Read the model definition and answer for the solid it produces. Units are mm, in the model's axes. Face numbers are marked on the shaded views. A direction names the side the tool comes from. Give positions to 0.01 mm unless a question says otherwise; leave off trailing zeros. Order: outer loops, then holes, each group sorted by start corner. A loop starts at its lowest first (then second) coordinate and runs counter-clockwise, first axis right, second up.
Item 1: A cutting plane is placed at B-B (x = 4.5). Write down the section's boundary in (y, z) (3 decimals), plus the area to 3 significant figures.
Item 2: A cutting plane is placed at C-C (z = -6). Write down the section's boundary in (x, y) (3 decimals).
Item 3: The mould has two halves that part along Y. Classify the marked faces 1, 2 and 3: +Y half, -Y half, draft (parallel to the pull), parting line (faces both ways), or undercut.
Item 4: Which of the six approach directions +Z, -Z, +X, -X, +Y, -Y give full straight-line access (tool end or side, diameter ignored) to the marked faces 4 and 5?
Item 5: A cutting plane is placed at A-A (y = 9.5). Write down the section's boundary in (x, z) (3 decimals).
Item 6: Given pin 1 Ø4.5 at (x, y) = (-23.241, 23.241) entering from -Z (3 decimals); pin 2 Ø1.7 at (x, y) = (23, -18) entering from +Z; pin 3 Ø3.5 at (x, y) = (22.86, 17.78) entering from +Z; pin 4 Ø4.5 at (x, y) = (-23.241, -23.241) entering from +Z (3 decimals), each flat-ended and moving along its own axis, determine where each tip first touches the part or whether it passes through.
Item 7: Find the intervals of material crossed by line 1 along X through (y, z) = (27.5, 0) (3 decimals); line 2 along X through (y, z) = (7, -1) (3 decimals); line 3 along Y through (x, z) = (1.5, 6) (3 decimals), in increasing order.
Item 8: A cutting plane is placed at D-D (x = 12.7). State how many separate pieces and enclosed holes the cut face has, plus the area to 3 significant figures.
from build123d import *

# Parameters (mm, degrees)
SKETCH1_W_MOCK_PCB_W                      = 57.15
SKETCH1_W_MOCK_PCB_H                      = 57.15
BOSS_EXTRUDE1_DEPTH                       = 6.985
CUT_EXTRUDE1_DEPTH                        = 2.54
CUT_EXTRUDE3_DEPTH                        = 3.8608
F_4_40_TAPPED_HOLE1_AT_2_COUNT            = 2
F_4_40_TAPPED_HOLE1_AT_2_PITCH            = 45.72
F_4_40_TAPPED_HOLE1_AT_3_COUNT            = 2
F_4_40_TAPPED_HOLE1_AT_3_PITCH            = 35.56
F_4_40_TAPPED_HOLE1_AT_4_COUNT            = 2
F_4_40_TAPPED_HOLE1_AT_4_PITCH            = 57.920911595
F_4_40_TAPPED_HOLE2_AT_2_COUNT            = 2
F_4_40_TAPPED_HOLE2_AT_2_PITCH            = 46.482
F_4_40_TAPPED_HOLE2_AT_3_COUNT            = 2
F_4_40_TAPPED_HOLE2_AT_3_PITCH            = 65.735474806
F_4_40_TAPPED_HOLE2_AT_4_COUNT            = 2
F_4_40_TAPPED_HOLE2_AT_4_PITCH            = 46.482
F_8_32_TAPPED_HOLE1_D                     = 4.1656
F_8_32_TAPPED_HOLE1_DEPTH                 = 4.953
F_8_32_TAPPED_HOLE1_CSINK_D               = 4.191
F_8_32_TAPPED_HOLE1_CSINK_ANGLE           = 90
F_8_32_TAPPED_HOLE1_ON_FACE_2_D           = 4.1656
F_8_32_TAPPED_HOLE1_ON_FACE_2_DEPTH       = 4.953
F_8_32_TAPPED_HOLE1_ON_FACE_2_CSINK_D     = 4.191
F_8_32_TAPPED_HOLE1_ON_FACE_2_CSINK_ANGLE = 90


with BuildPart() as part:
    # Sketch1 w/mock PCB → Boss-Extrude1 (new body, symmetric)
    with BuildSketch(Plane.XY):
        Rectangle(SKETCH1_W_MOCK_PCB_W, SKETCH1_W_MOCK_PCB_H)
        with BuildLine():
            Line((20.32, 17.78), (20.32, 20.447))
            ThreePointArc((20.32, 20.447), (19.39006403, 22.69206403), (17.145, 23.622))
            Line((17.145, 23.622), (-17.145, 23.622))
            ThreePointArc((-17.145, 23.622), (-19.39006403, 22.69206403), (-20.32, 20.447))
            Line((-20.32, 20.447), (-20.32, 17.78))
            ThreePointArc((-20.32, 17.78), (-21.044102303, 16.004017017), (-22.803555556, 15.240627238))
            ThreePointArc((-22.803555556, 15.240627238), (-25.002872121, 14.286390014), (-25.908, 12.066411285))
            Line((-25.908, 12.066411285), (-25.908, -12.066411285))
            ThreePointArc((-25.908, -12.066411285), (-25.002872121, -14.286390014), (-22.803555556, -15.240627238))
            ThreePointArc((-22.803555556, -15.240627238), (-21.044102303, -16.004017017), (-20.32, -17.78))
            Line((-20.32, -17.78), (-20.32, -20.447))
            ThreePointArc((-20.32, -20.447), (-19.39006403, -22.69206403), (-17.145, -23.622))
            Line((-17.145, -23.622), (17.145, -23.622))
            ThreePointArc((17.145, -23.622), (19.39006403, -22.69206403), (20.32, -20.447))
            Line((20.32, -20.447), (20.32, -17.78))
            ThreePointArc((20.32, -17.78), (21.044102303, -16.004017017), (22.803555556, -15.240627238))
            ThreePointArc((22.803555556, -15.240627238), (25.002872121, -14.286390014), (25.908, -12.066411285))
            Line((25.908, -12.066411285), (25.908, 12.066411285))
            ThreePointArc((25.908, 12.066411285), (25.002872121, 14.286390014), (22.803555556, 15.240627238))
            ThreePointArc((22.803555556, 15.240627238), (21.044102303, 16.004017017), (20.32, 17.78))
        make_face(mode=Mode.SUBTRACT)
    extrude(amount=BOSS_EXTRUDE1_DEPTH, both=True)

    # Sketch2 → Cut-Extrude1 (cut)
    with BuildSketch(Plane.XY.offset(6.985)):
        with BuildLine():
            Line((-23.876, 27.051), (23.876, 27.051))
            ThreePointArc((23.876, 27.051), (26.12106403, 26.12106403), (27.051, 23.876))
            Line((27.051, 23.876), (27.051, -23.876))
            ThreePointArc((27.051, -23.876), (26.12106403, -26.12106403), (23.876, -27.051))
            Line((23.876, -27.051), (-23.876, -27.051))
            ThreePointArc((-23.876, -27.051), (-26.12106403, -26.12106403), (-27.051, -23.876))
            Line((-27.051, -23.876), (-27.051, 23.876))
            ThreePointArc((-27.051, 23.876), (-26.12106403, 26.12106403), (-23.876, 27.051))
        make_face()
    cut_extrude1 = extrude(amount=-CUT_EXTRUDE1_DEPTH, mode=Mode.SUBTRACT)

    # Mirror1: Cut-Extrude1 across plane
    add(cut_extrude1.mirror(Plane.XY), mode=Mode.SUBTRACT)

    # Sketch4 → Cut-Extrude3 (cut)
    with BuildSketch(Plane.XY.offset(4.445)):
        with BuildLine():
            Line((-20.32, 17.78), (-20.32, 20.447))
            ThreePointArc((-20.32, 20.447), (-20.314259086, 20.637845079), (-20.297057106, 20.828))
            Line((-20.297057106, 20.828), (-22.733, 20.828))
            ThreePointArc((-22.733, 20.828), (-24.97806403, 19.89806403), (-25.908, 17.653))
            Line((-25.908, 17.653), (-25.908, 12.066411285))
            ThreePointArc((-25.908, 12.066411285), (-25.002872121, 14.286390014), (-22.803555556, 15.240627238))
            ThreePointArc((-22.803555556, 15.240627238), (-21.044102303, 16.004017017), (-20.32, 17.78))
        make_face()
        with BuildLine():
            Line((25.908, -12.066411285), (25.908, -17.653))
            ThreePointArc((25.908, -17.653), (24.97806403, -19.89806403), (22.733, -20.828))
            Line((22.733, -20.828), (20.297057106, -20.828))
            ThreePointArc((20.297057106, -20.828), (20.314259086, -20.637845079), (20.32, -20.447))
            Line((20.32, -20.447), (20.32, -17.78))
            ThreePointArc((20.32, -17.78), (21.044102303, -16.004017017), (22.803555556, -15.240627238))
            ThreePointArc((22.803555556, -15.240627238), (25.002872121, -14.286390014), (25.908, -12.066411285))
        make_face()
        with BuildLine():
            Line((-25.908, -12.066411285), (-25.908, -17.653))
            ThreePointArc((-25.908, -17.653), (-24.97806403, -19.89806403), (-22.733, -20.828))
            Line((-22.733, -20.828), (-20.297057106, -20.828))
            ThreePointArc((-20.297057106, -20.828), (-20.314259086, -20.637845079), (-20.32, -20.447))
            Line((-20.32, -20.447), (-20.32, -17.78))
            ThreePointArc((-20.32, -17.78), (-21.044102303, -16.004017017), (-22.803555556, -15.240627238))
            ThreePointArc((-22.803555556, -15.240627238), (-25.002872121, -14.286390014), (-25.908, -12.066411285))
        make_face()
        with BuildLine():
            Line((20.297057106, 20.828), (22.733, 20.828))
            ThreePointArc((22.733, 20.828), (24.97806403, 19.89806403), (25.908, 17.653))
            Line((25.908, 17.653), (25.908, 12.066411285))
            ThreePointArc((25.908, 12.066411285), (25.002872121, 14.286390014), (22.803555556, 15.240627238))
            ThreePointArc((22.803555556, 15.240627238), (21.044102303, 16.004017017), (20.32, 17.78))
            Line((20.32, 17.78), (20.32, 20.447))
            ThreePointArc((20.32, 20.447), (20.314259086, 20.637845079), (20.297057106, 20.828))
        make_face()
    extrude(amount=-CUT_EXTRUDE3_DEPTH, mode=Mode.SUBTRACT)

    # Sketch11 → #4-40 Tapped Hole1 (revolve, cut)
    with BuildSketch(Plane(origin=(22.86, 17.78, 0.5842), x_dir=(0, -1, 0), z_dir=(1, 0, 0))):
        Polygon((0, 0), (0, 5.0292), (1.4351, 5.0292), (1.4224, 5.0165), (1.4224, 0.0127), (1.4351, 0), align=None)
    f_4_40_tapped_hole1 = revolve(axis=Axis((22.86, 17.78, 6.9342), (0, 0, -1)), mode=Mode.SUBTRACT)

    # #4-40 Tapped Hole1 at 2: #4-40 Tapped Hole1 ×2
    with Locations(*[(-i * F_4_40_TAPPED_HOLE1_AT_2_PITCH, 0, 0) for i in range(1, F_4_40_TAPPED_HOLE1_AT_2_COUNT)]):
        add(f_4_40_tapped_hole1, mode=Mode.SUBTRACT)

    # #4-40 Tapped Hole1 at 3: #4-40 Tapped Hole1 ×2
    with Locations(*[(0, -i * F_4_40_TAPPED_HOLE1_AT_3_PITCH, 0) for i in range(1, F_4_40_TAPPED_HOLE1_AT_3_COUNT)]):
        add(f_4_40_tapped_hole1, mode=Mode.SUBTRACT)

    # #4-40 Tapped Hole1 at 4: #4-40 Tapped Hole1 ×2
    with Locations(*[Vector(-0.789352217, -0.613940614, 0) * (i * F_4_40_TAPPED_HOLE1_AT_4_PITCH) for i in range(1, F_4_40_TAPPED_HOLE1_AT_4_COUNT)]):
        add(f_4_40_tapped_hole1, mode=Mode.SUBTRACT)

    # Sketch22 → #4-40 Tapped Hole2 (revolve, cut)
    with BuildSketch(Plane(origin=(-23.241, 23.241, 4.445), x_dir=(0, -1, 0), z_dir=(1, 0, 0))):
        Polygon((0, 0), (0, 8.89), (1.4351, 8.89), (1.4224, 8.8773), (1.4224, 0.0127), (1.4351, 0), align=None)
    f_4_40_tapped_hole2 = revolve(axis=Axis((-23.241, 23.241, 10.795), (0, 0, -1)), mode=Mode.SUBTRACT)

    # #4-40 Tapped Hole2 at 2: #4-40 Tapped Hole2 ×2
    with Locations(*[(i * F_4_40_TAPPED_HOLE2_AT_2_PITCH, 0, 0) for i in range(1, F_4_40_TAPPED_HOLE2_AT_2_COUNT)]):
        add(f_4_40_tapped_hole2, mode=Mode.SUBTRACT)

    # #4-40 Tapped Hole2 at 3: #4-40 Tapped Hole2 ×2
    with Locations(*[Vector(0.707106781, -0.707106781, 0) * (i * F_4_40_TAPPED_HOLE2_AT_3_PITCH) for i in range(1, F_4_40_TAPPED_HOLE2_AT_3_COUNT)]):
        add(f_4_40_tapped_hole2, mode=Mode.SUBTRACT)

    # #4-40 Tapped Hole2 at 4: #4-40 Tapped Hole2 ×2
    with Locations(*[(0, -i * F_4_40_TAPPED_HOLE2_AT_4_PITCH, 0) for i in range(1, F_4_40_TAPPED_HOLE2_AT_4_COUNT)]):
        add(f_4_40_tapped_hole2, mode=Mode.SUBTRACT)

    # #8-32 Tapped Hole1
    with Locations(Plane(origin=(-12.7, 28.575, 0), x_dir=(0, 0, 1), z_dir=(0, 1, 0))):
        with Locations((0, 0), (0, 25.4), (0, 12.7)):
            CounterSinkHole(F_8_32_TAPPED_HOLE1_D / 2, F_8_32_TAPPED_HOLE1_CSINK_D / 2, depth=F_8_32_TAPPED_HOLE1_DEPTH, counter_sink_angle=F_8_32_TAPPED_HOLE1_CSINK_ANGLE)

    # #8-32 Tapped Hole1 on face 2
    with Locations(Plane(origin=(12.7, -28.575, 0), x_dir=(0, 0, -1), z_dir=(0, -1, 0))):
        with Locations((0, 0), (0, -12.7), (0, -25.4)):
            CounterSinkHole(F_8_32_TAPPED_HOLE1_ON_FACE_2_D / 2, F_8_32_TAPPED_HOLE1_ON_FACE_2_CSINK_D / 2, depth=F_8_32_TAPPED_HOLE1_ON_FACE_2_DEPTH, counter_sink_angle=F_8_32_TAPPED_HOLE1_ON_FACE_2_CSINK_ANGLE)


solid = part.part
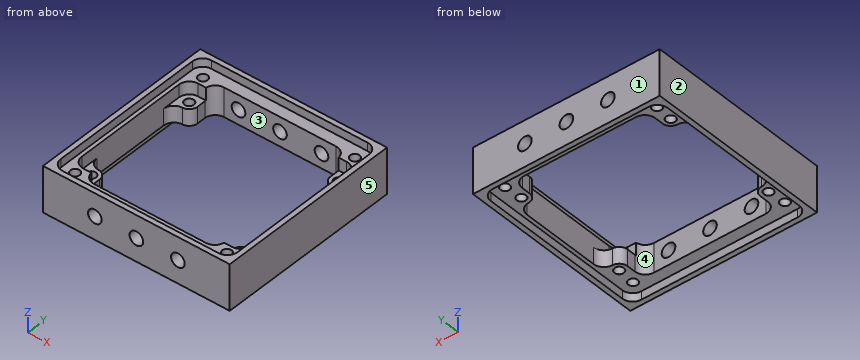
Response values:
1. outline: (-28.575, -6.985) - (-27.051, -6.985) - (-27.051, -4.445) - (-23.622, -4.445) - (-23.622, 4.445) - (-27.051, 4.445) - (-27.051, 6.985) - (-28.575, 6.985) - close; (23.622, -4.445) - (27.051, -4.445) - (27.051, -6.985) - (28.575, -6.985) - (28.575, 6.985) - (27.051, 6.985) - (27.051, 4.445) - (23.622, 4.445) - close
1. area: 104 mm2
2. outline: (-28.575, -28.575) - (28.575, -28.575) - (28.575, 28.575) - (-28.575, 28.575) - close; hole (-27.051, -23.876) arc R3.175 ccw to (-23.876, -27.051) - (23.876, -27.051) arc R3.175 ccw to (27.051, -23.876) - (27.051, 23.876) arc R3.175 ccw to (23.876, 27.051) - (-23.876, 27.051) arc R3.175 ccw to (-27.051, 23.876) - close
3. face 1: +Y half
3. face 2: draft
3. face 3: undercut
4. face 4: +Z, -Z
4. face 5: +Z, -Z, +X, +Y, -Y
5. outline: (-28.575, -6.985) - (-27.051, -6.985) - (-27.051, -4.445) - (-25.908, -4.445) - (-25.908, 4.445) - (-27.051, 4.445) - (-27.051, 6.985) - (-28.575, 6.985) - close; (25.908, -4.445) - (27.051, -4.445) - (27.051, -6.985) - (28.575, -6.985) - (28.575, 6.985) - (27.051, 6.985) - (27.051, 4.445) - (25.908, 4.445) - close
6. pin 1: stops at z = -4.445
6. pin 2: passes through
6. pin 3: stops at z = 0.58
6. pin 4: stops at z = 4.445
7. line 1: x = -28.575 to -14.783, -10.617 to -2.083, 2.083 to 10.617, 14.783 to 28.575
7. line 2: x = -28.575 to -25.908, 25.908 to 28.575
7. line 3: y = -28.575 to -27.051, 27.051 to 28.575
8. separate pieces: 4
8. enclosed holes: 0
8. area: 62.3 mm2
